Work out the finished part from the listing and answer in its coordinate system (mm). Give positions to 0.01 mm unless a question says otherwise; leave off trailing zeros. Order: outer loops, then holes, each group sorted by start corner. A loop starts at its lowest first (then second) coordinate and runs counter-clockwise, first axis right, second up.
```python
from build123d import *

# Parameters (mm, degrees)
CROQUIS1_W              = 40
CROQUIS1_H              = 40
CROQUIS1_R              = 4.5
SALIENTE_EXTRUIR1_DEPTH = 4.5
CHAFL_N1_SIZE           = 1


with BuildPart() as part:
    # Croquis1 → Saliente-Extruir1 (new body)
    with BuildSketch(Plane.XY):
        Rectangle(CROQUIS1_W, CROQUIS1_H)
        Circle(CROQUIS1_R, mode=Mode.SUBTRACT)
    extrude(amount=SALIENTE_EXTRUIR1_DEPTH)

    # Chaflán1
    chafl_n1_edges = [part.edges().sort_by_distance(p)[0] for p in [
        (-20, 0, 4.5),
        (0, -20, 4.5),
        (20, 0, 4.5),
        (20, -20, 2.25),
        (-20, -20, 2.25),
        (-20, 20, 2.25),
        (20, 20, 2.25),
        (0, 20, 4.5),
    ]]
    chamfer(chafl_n1_edges, length=CHAFL_N1_SIZE)


solid = part.part
```
1. Straight lines are drawn through the part: probe 1 along Y at (x, z) = (0, 1.35); probe 2 along Y at (x, z) = (-1.5, 0.9); probe 3 along X at (y, z) = (-3.5, 0.7). For each, find the intervals that lie inside material, in ascending order.
Findings below:
probe 1: y = -20 to -4.5, 4.5 to 20
probe 2: y = -20 to -4.24, 4.24 to 20
probe 3: x = -20 to -2.83, 2.83 to 20
2. The mould has two halves that part along Y. Classify faces 1 (the face through (0, 5, 0)), 2 (the face through (-0.3, -19.5, 4)), 3 (the face through (-0.59, 4.46, 2.22)), 4 (the face through (-19.5, 19.5, 1.7)): pulls with the +Y half, pulls with the -Y half, needs draft (parallel to the pull), parting line crosses it, or undercut.
Findings below:
face 1: needs draft
face 2: pulls with the -Y half
face 3: undercut
face 4: pulls with the +Y half
3. The part is cut by section A-A (y = 0). Write down the section's boundary in (x, z), then the cut area to 4 significant figures.
Findings below:
outline: (-20, 0) - (-4.5, 0) - (-4.5, 4.5) - (-19, 4.5) - (-20, 3.5) - close; (4.5, 0) - (20, 0) - (20, 3.5) - (19, 4.5) - (4.5, 4.5) - close
area: 138.5 mm2
4. The part is cut by section B-B (z = 1.75). Write down the section's boundary in (x, y).
Findings below:
outline: (-20, -19) - (-19, -20) - (19, -20) - (20, -19) - (20, 19) - (19, 20) - (-19, 20) - (-20, 19) - close; hole circle Ø9 at (0, 0)
5. Given P1, Ø6, axis at x = -3, y = 6, coming from the -Z side, flat-ended and moving along its own axis, determine where the tip first touches the part or whether it passes through.
Findings below:
P1: stops at z = 0
